Part model, mm, in its own coordinate system. Face numbers are marked on the shaded views. A direction names the side the tool comes from. Give positions to 0.01 mm unless a question says otherwise; leave off trailing zeros. Order: outer loops, then holes, each group sorted by start corner. A loop starts at its lowest first (then second) coordinate and runs counter-clockwise, first axis right, second up. Notation, with made-up numbers: (17, 47.5) - (52, 47.5) arc R17 cw to (52, 58.5) - close; hole circle Ø6 at (-16.5, 63.25). An arc over 180 degrees is marked (long way). Use a Markdown table: item, result. Add a question column.
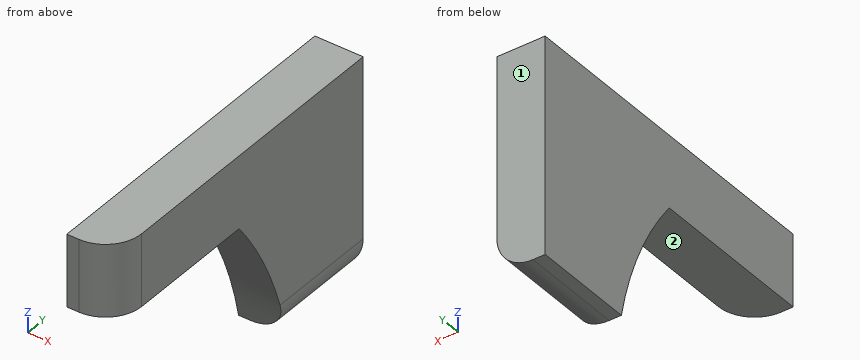
from build123d import *

# Parameters (mm, degrees)
BOX092_W          = 2
BOX092_H          = 14
BOX092_DEPTH      = 3
FILLET012_R       = 1.5
CYLINDER046_R     = 15
CYLINDER046_DEPTH = 4
BOX094_W          = 2
BOX094_H          = 10
BOX094_DEPTH      = 6
FILLET058_R       = 1.5


with BuildPart() as fillet012:
    # Box092 → Box092 (new body)
    with BuildSketch(Plane(origin=(31, 36, -6), x_dir=(1, 0, 0), z_dir=(0, 0, 1))):
        with Locations((1, 7)):
            Rectangle(BOX092_W, BOX092_H)
    extrude(amount=BOX092_DEPTH)

    # Fillet012
    fillet012_edges = [fillet012.edges().sort_by_distance(p)[0] for p in [
        (33, 36, -4.5),
    ]]
    fillet(fillet012_edges, radius=FILLET012_R)


with BuildPart() as cylinder130:
    # Cylinder046 → Cylinder046 (new body)
    with BuildSketch(Plane(origin=(30, 31, -15), x_dir=(0, 0, -1), z_dir=(1, 0, 0))):
        Circle(CYLINDER046_R)
    extrude(amount=CYLINDER046_DEPTH)


with BuildPart() as fusion073:
    # Box094 → Box094 (new body)
    with BuildSketch(Plane(origin=(31, 40, -12), x_dir=(1, 0, 0), z_dir=(0, 0, 1))):
        with Locations((1, 5)):
            Rectangle(BOX094_W, BOX094_H)
    extrude(amount=BOX094_DEPTH)

    # Cut121: cut Cylinder130
    add(cylinder130.part, mode=Mode.SUBTRACT)

    # Fillet058
    fillet058_edges = [fusion073.edges().sort_by_distance(p)[0] for p in [
        (33, 47.848469, -12),
    ]]
    fillet(fillet058_edges, radius=FILLET058_R)

    # Fusion073: union Fillet012
    add(fillet012.part)


solid = fusion073.part
1. Pin check, flat tip, straight feed: P1, Ø0.6, axis at x = 32, y = 38, coming from the -Z side. Stop position of the tip, or through.
2. Cut at A-A (x = 31.3). Write the cut outline in (y, z).
3. Drill centre lines: probe 1 along Z at (x, y) = (32.95, 40.75); probe 2 along Y at (x, z) = (32.65, -5); probe 3 along Y at (x, z) = (31.8, -8.5). Where is each one in solid material? Low to high. Write a range as [from, to].
4. Cut at D-D (x = 32.5). Write the cut outline in (y, z), plus the area to 3 significant figures.
5. Cut at C-C (z = -4). Write the cut outline in (x, y), plus the area to 3 significant figures.
6. Tool access for the marked faces 1 and 2: list every direction of +Z, -Z, +X, -X, +Y, -Y with a clear straight run to the whole face (end or side of a thin tool).
7. Cut at B-B (y = 48.25). Write the cut outline in (x, z), plus the area to 3 significant figures.
Responses:
| question | item | result |
|---|---|---|
| 1 | P1 | stops at z = -6 |
| 2 | outline | (36, -6) - (43, -6) arc R15 cw to (45.7, -12) - (50, -12) - (50, -3) - (36, -3) - close |
| 3 | probe 1 | z = [-6, -3] |
| 3 | probe 2 | y = [36.54, 50] |
| 3 | probe 3 | y = [44.52, 50] |
| 4 | outline | (36.38, -6) - (43, -6) arc R15 cw to (45.61, -11.62) - (50, -11.62) - (50, -3) - (36.38, -3) - close |
| 4 | area | 71.5 mm² |
| 5 | outline | (31, 36) - (31.5, 36) arc R1.5 ccw to (33, 37.5) - (33, 50) - (31, 50) - close |
| 5 | area | 27.5 mm² |
| 6 | face 1 | +Z, -Z, +X, -X, +Y |
| 6 | face 2 | -Z, +X, -X, -Y |
| 7 | outline | (31, -12) - (31.5, -12) arc R1.5 ccw to (33, -10.5) - (33, -3) - (31, -3) - close |
| 7 | area | 17.5 mm² |
